Part model, mm, in its own coordinate system. Face numbers are marked on the shaded views. A direction names the side the tool comes from. Round coordinates to 2 decimals unless told otherwise and drop trailing zeros. Loops run counter-clockwise (first coordinate to the right, second up) from the corner with the lowest first, then second, coordinate; pieces in that order, holes last. Notation, with made-up numbers: M 73.25,22 L 95.25,22 A28 cw 95.25,51 Z; hole C 85.5,14.25 d9. An arc over 180 degrees is marked long. Answer as CSV lines item,"result". Start each with the question number.
Item 1: Band-saw the part on A-A (z = 20). Give the cut face in (x, y), and give its area (3 significant figures).
Item 2: Band-saw the part on D-D (z = 24). Give the cut face in (x, y), and give its area (3 significant figures).
Item 3: Which spindle directions (+Z, -Z, +X, -X, +Y, -Y) get a long thin tool onto all of the face, cutting with end or side? Do the marked faces 1, 2 and 3. Say none if no direction does.
Item 4: Band-saw the part on C-C (x = 3.5). Give the cut face in (y, z).
Item 5: Band-saw the part on B-B (y = 6). Give the cut face in (x, z), and give its area (3 significant figures).
Item 6: Drop flat-ended pins along their axis: pin 1 Ø3.5 at (x, z) = (9, 29.5) entering from -Y; pin 2 Ø5 at (y, z) = (5, 28) entering from +X; pin 3 Ø6 at (x, y) = (-4.5, 6) entering from -Z; pin 4 Ø2 at (x, y) = (-17.5, 9.5) entering from +Z. Give the stop position or say it passes through.
Item 7: Wall check: line 1 (X direction, y = 8, z = 9.5); line 2 (X direction, y = 1.75, z = 29.5). Give the ranges that are in metal, low to high.
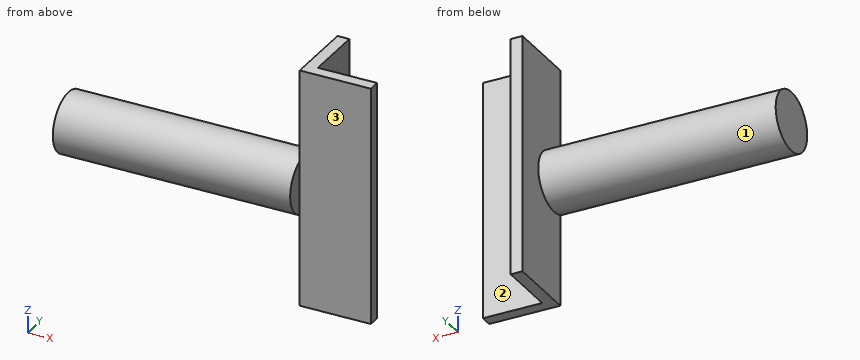
```python
from build123d import *

# Parameters (mm, degrees)
BOSS_EXTRU_1_DEPTH = 40
ESQUISSE2_R        = 5
BOSS_EXTRU_2_DEPTH = 40


with BuildPart() as part:
    # Esquisse1 → Boss.-Extru.1 (new body)
    with BuildSketch(Plane.XY):
        Polygon((0, 0), (0, 12), (2, 12), (2, 2), (12, 2), (12, 0), align=None)
    extrude(amount=BOSS_EXTRU_1_DEPTH)

    # Esquisse2 → Boss.-Extru.2 (add)
    with BuildSketch(Plane.ZY):
        with Locations(Location((20, 2, 0), (0, 0, 203.578178478))):
            Circle(ESQUISSE2_R)
    extrude(amount=BOSS_EXTRU_2_DEPTH)


solid = part.part
```
Answer block:
1,outline,"M -40,-3 L 0,-3 L 0,0 L 12,0 L 12,2 L 2,2 L 2,12 L 0,12 L 0,7 L -40,7 Z"
1,area,"444 mm^2"
2,outline,"M -40,-1 L 0,-1 L 0,0 L 12,0 L 12,2 L 2,2 L 2,12 L 0,12 L 0,5 L -40,5 Z"
2,area,"284 mm^2"
3,face 1,"-X"
3,face 2,"+Z, -Z, +X, +Y"
3,face 3,"+Z, -Z, +X, -Y"
4,outline,"M 0,0 L 2,0 L 2,40 L 0,40 Z"
5,outline,"M -40,17 L 0,17 L 0,0 L 2,0 L 2,40 L 0,40 L 0,23 L -40,23 Z"
5,area,"320 mm^2"
6,pin 1,"stops at y = 0"
6,pin 2,"stops at x = 2"
6,pin 3,"stops at z = 15.1"
6,pin 4,"passes through"
7,line 1,"x = 0 to 2"
7,line 2,"x = 0 to 12"
